```python
from build123d import *

# Parameters (mm, degrees)
ESBO_O5_R             = 10.153899328
CORTE_EXTRUS_O1_DEPTH = 7
CHANFRO1_SIZE         = 1
FILETE1_R             = 1
CHANFRO2_SIZE         = 2
CHANFRO2_SIZE2        = 2.383507185


with BuildPart() as part:
    # Esboço4 → Revolução1 (revolve)
    with BuildSketch(Plane(origin=(0, 0, 0), x_dir=(0, 0, -1), z_dir=(1, 0, 0)), mode=Mode.PRIVATE) as revolu_o1_sk:
        Polygon((-4.9, 0), (-4.9, 20), (-2.5, 20), (-2.5, 18), (-1.5, 16.267949192), (0, 16.267949192), (1.5, 16.267949192), (2.5, 18), (2.5, 20), (4.9, 20), (4.9, 0), align=None)
    revolve(revolu_o1_sk.sketch.rotate(Axis((0, -1.5, 9.058267024), (0, 0, -1)), 90), axis=Axis((0, -1.5, 9.058267024), (0, 0, -1)))

    # Esboço5 → Corte-extrusão1 (cut)
    with BuildSketch(Plane.XY.offset(4.9)):
        with Locations((0, -1.5)):
            Circle(ESBO_O5_R)
    extrude(amount=-CORTE_EXTRUS_O1_DEPTH, mode=Mode.SUBTRACT)

    # Chanfro1
    chanfro1_edges = [part.edges().sort_by_distance(p)[0] for p in [
        (-10.153899328, -1.5, 4.9),
    ]]
    chamfer(chanfro1_edges, length=CHANFRO1_SIZE)

    # Filete1
    filete1_edges = [part.edges().sort_by_distance(p)[0] for p in [
        (-10.153899328, -1.5, -2.1),
    ]]
    fillet(filete1_edges, radius=FILETE1_R)

    # Chanfro2
    chanfro2_edges = [part.edges().sort_by_distance(p)[0] for p in [
        (-1.5, -1.5, -4.9),
    ]]
    chanfro2_side = [part.faces().sort_by_distance(p)[0] for p in [
        (-1.5, -1.5, -3.5),
    ]]
    chamfer(chanfro2_edges, length=CHANFRO2_SIZE, length2=CHANFRO2_SIZE2, reference=chanfro2_side[0])


solid = part.part
```
Here's how the part is built. I have some questions about the finished solid (model axes, mm). A direction names the side the tool comes from. Give positions to 0.01 mm unless a question says otherwise; leave off trailing zeros. Write each loop counter-clockwise with the first axis right and the second up, starting at its lowest first coordinate (ties: lowest second). Pieces come first, ordered by that corner, then holes. Notation, with made-up numbers: M -22,-38.75 L 9,-38.75 A24 cw 9,-21.75 Z; hole C 27,53.5 d1. An arc over 180 degrees is marked long. Put each result on its own line as item: value. Start each with the question number.
Item 1: Will these pins go through, and if not, where does the flat tip stop? pin 1 (1.5 mm diameter, centred on y = 1.5, z = -4, fed in from +X); pin 2 (5.5 mm diameter, centred on x = 1, y = -0.5, fed in from +Z); pin 3 (5 mm diameter, centred on x = -3, z = 3.5, fed in from +Y).
Item 2: Thinking about a two-plate mould opening in Y: for faces 4 (the cylindrical face through (1.43, -1.95, -2.49)), 5 (the cylindrical face through (-17.75, -2.28, 0.02)), 6 (the flat face through (4.5, -1.8, -4.9)), which applies, +Y half, -Y half, draft (parallel to the pull), parting line (faces both ways), or undercut?
Item 3: If we section it at D-D, the plane z = 1: Write out the boundary of the cut face in (x, y), then the cut area to 3 significant figures.
Item 4: If we section it at C-C, the plane z = 3.25: Write out the boundary of the cut face in (x, y).
Item 5: On a 3-axis mill with a long thin cutter (end or side, diameter ignored), from which of +Z, -Z, +X, -X, +Y, -Y can I reach the whole of each face in a straight line? I mean faces 1 (the cylindrical face through (4.7, -10.5, 1.4)), 2 (the flat face through (-5, 18, -2.5)), 3 (the cylindrical face through (-2.799, -22.817, -3.717)). Say none if no direction works.
Item 6: I need wall thicknesses on L1, parallel to Z at x = 18, y = -9; L2, parallel to Y at x = 0, z = -2.55; L3, parallel to Z at x = 10.5, y = -17.5. Which ranges of each line are inside material? Lowest first, please. Write a range as from..to.
Values:
1. pin 1: x = 21.38
1. pin 2: z = -2.1
1. pin 3: y = 19.99
2. face 4: undercut
2. face 5: parting line
2. face 6: draft
3. outline: C 0,-1.5 d35.54; hole C 0,-1.5 d20.31
3. area: 668 mm²
4. outline: C 0,-1.5 d43; hole C 0,-1.5 d20.31
5. face 1: +Z
5. face 2: none
5. face 3: +Z, -Z
6. L1: -4.9..-2.5, 2.5..4.9
6. L2: -23..-3, 0..20
6. L3: -4.9..-2.29, 2.29..4.9
